Autodesk Inventor part; units mm, degrees
ref_plane "YZ Plane" through (0, 0, 0) normal (1, 0, 0) x (0, 1, 0)
ref_plane "XZ Plane" through (0, 0, 0) normal (0, 1, 0) x (-1, 0, 0)
ref_plane "XY Plane" through (0, 0, 0) normal (0, 0, 1) x (1, 0, 0)
sketch "Esboço1" plane through (0, 0, 0) normal (0, 0, 1) x (1, 0, 0)
  line L0 (0, 0) -> (0, 25)
  line L1 (0, 25) -> (15, 25)
  line L2 (15, 25) -> (15, 17.5)
  line L3 (15, 17.5) -> (50, 17.5)
  line L4 (50, 17.5) -> (50, 10)
  line L5 (50, 10) -> (80, 10)
  line L6 (80, 10) -> (80, 0)
  line L7 (80, 0) -> (0, 0)
  dimension "d0" = 50
  dimension "d1" = 35
  dimension "d2" = 20
  dimension "d3" = 15
  dimension "d4" = 65
  dimension "d5" = 30
revolve "Revolução1" add sketch "Esboço1" angle 360 about axis through (80, 0, 0) along (-1, 0, 0)
fillet "Arredondamento1" radius 3 2 edges at (15, -17.5, 0) (50, -10, 0)
chamfer "Chanfro1" distance 2 angle 45 1 edges at (80, -10, 0)
chamfer "Chanfro2" distance 5 angle 45 1 edges at (0, -25, 0)
sketch "Esboço2" plane through (80, 0, 0) normal (1, 0, 0) x (0, 0, -1)
  circle A0 centre (0, 0) radius 10
hole "Furo1" at (80, 0, 0) direction (-1, 0, 0) diameter 10 end through all
properties part number "3D Model"
Geometry check sheet. Reference: the model listing, model coordinates, mm. A direction names the side the tool comes from. Give positions to 0.01 mm unless a question says otherwise; leave off trailing zeros. Loops run counter-clockwise (first coordinate to the right, second up) from the corner with the lowest first, then second, coordinate; pieces in that order, holes last. Notation, with made-up numbers: M 25.25,-13.75 L 39.25,-13.75 A24 cw 39.25,12.25 Z; hole C 59.25,-1.75 d11. An arc over 180 degrees is marked long. Answer as CSV lines item,"result".
Item 1: Access from +Z, -Z, +X, -X, +Y, -Y to the whole of each face (thin tool, end or side, straight path). Record for faces 4 (the cylindrical face through (10.07, 23.846, 7.509)), 5 (the flat face through (50, -3, -13)).
Values:
face 4,"+X, -X"
face 5,"+X"
Item 2: Cross-section at C-C on x = 20. Record the cut outline in (y, z).
Values:
outline,"C 0,0 d35; hole C 0,0 d10"
Item 3: Material ranges on line 1 (Y direction, x = 36.5, z = 0); line 2 (Z direction, x = 58, y = 0); line 3 (X direction, y = -14, z = -7.5), recorded low to high.
Values:
line 1,"y = -17.5 to -5, 5 to 17.5"
line 2,"z = -10 to -5, 5 to 10"
line 3,"x = 0 to 50"
Item 4: Cross-section at A-A on z = 0. Record the cut outline in (x, y).
Values:
outline,"M 0,-20 L 5,-25 L 15,-25 L 15,-20.5 A3 cw 18,-17.5 L 50,-17.5 L 50,-13 A3 cw 53,-10 L 78,-10 L 80,-8 L 80,-5 L 0,-5 Z; M 0,5 L 80,5 L 80,8 L 78,10 L 53,10 A3 cw 50,13 L 50,17.5 L 18,17.5 A3 cw 15,20.5 L 15,25 L 5,25 L 0,20 Z"
Item 5: Release check for a two-part mould opening along Y. For faces 1 (the cylindrical face through (39.44, 4.88, 1.08)), 2 (the flat face through (80, -0.1, 5.2)), 3 (the conical face through (79.87, -1.06, -8.06)) record: pulls with the +Y half, pulls with the -Y half, needs draft (parallel to the pull), parting line crosses it, or undercut.
Values:
face 1,"undercut"
face 2,"needs draft"
face 3,"parting line crosses it"
Item 6: Depth check by flat-ended pin: P1, Ø1, axis at y = -18, z = 12.5, coming from the +X side; P2, Ø10, axis at y = -13.5, z = -6, coming from the -X side; P3, Ø6, axis at x = 8.5, y = -17.5, coming from the +Z side; P4, Ø2, axis at x = 41.5, z = 10.5, coming from the +Y side. Enter the tip coordinate at first touch or a pass-through.
Values:
P1,"stops at x = 15"
P2,"stops at x = 0"
P3,"stops at z = 20.37"
P4,"stops at y = 14.7"
Item 7: Cross-section at D-D on x = 74.5. Record the cut outline in (y, z).
Values:
outline,"C 0,0 d20; hole C 0,0 d10"
